Here's how the part is built. I have some questions about the finished solid (model axes, mm). A direction names the side the tool comes from. Round coordinates to 2 decimals unless told otherwise and drop trailing zeros. Loops run counter-clockwise (first coordinate to the right, second up) from the corner with the lowest first, then second, coordinate; pieces in that order, holes last. Notation, with made-up numbers: M 51.5,67.25 L 66.5,67.25 A19 cw 66.5,89.25 Z; hole C 53,79.5 d5. An arc over 180 degrees is marked long. Use a Markdown table: item, result.
```python
from build123d import *

# Parameters (mm, degrees)
BOSS_EXTRUDE1_DEPTH     = 12.7
SKETCH3_W               = 102.447825146
SKETCH3_H               = 31.827107341
BOSS_EXTRUDE2_DEPTH     = 88.9
SKETCH4_R               = 63.5
PILOT_DIA_DEPTH         = 3.175
F_1_2_20_TAPPED_HOLE2_D = 11.50874
CIRPATTERN2_COUNT       = 4


with BuildPart() as part:
    # Sketch1 → Base-Revolve (revolve)
    with BuildSketch(Plane.XY, mode=Mode.PRIVATE) as base_revolve_sk:
        with BuildLine():
            Line((0, 0), (0, 12.7))
            Line((0, 12.7), (-50.8, 12.7))
            Line((-50.8, 12.7), (-50.8, 69.85))
            Line((-50.8, 69.85), (-266.7, 69.85))
            Line((-266.7, 69.85), (-266.7, 76.2))
            Line((-266.7, 76.2), (-279.4, 76.2))
            ThreePointArc((-279.4, 76.2), (-297.360512242, 68.760512242), (-304.8, 50.8))
            Line((-304.8, 50.8), (-304.8, 0))
            Line((-304.8, 0), (0, 0))
        make_face()
    revolve(base_revolve_sk.sketch.rotate(Axis((0, 0, 0), (1, 0, 0)), 90), axis=Axis((0, 0, 0), (1, 0, 0)))

    # Sketch2 → Boss-Extrude1 (add)
    with BuildSketch(Plane(origin=(-50.8, 0, 0), x_dir=(0, 0, -1), z_dir=(1, 0, 0))):
        with BuildLine():
            Line((74.6125, -58.7375), (74.6125, 58.7375))
            ThreePointArc((74.6125, 58.7375), (69.962820151, 69.962820151), (58.7375, 74.6125))
            Line((58.7375, 74.6125), (-58.7375, 74.6125))
            ThreePointArc((-58.7375, 74.6125), (-69.962820151, 69.962820151), (-74.6125, 58.7375))
            Line((-74.6125, 58.7375), (-74.6125, -58.7375))
            ThreePointArc((-74.6125, -58.7375), (-69.962820151, -69.962820151), (-58.7375, -74.6125))
            Line((-58.7375, -74.6125), (58.7375, -74.6125))
            ThreePointArc((58.7375, -74.6125), (69.962820151, -69.962820151), (74.6125, -58.7375))
        make_face()
    extrude(amount=-BOSS_EXTRUDE1_DEPTH)

    # Sketch3 → Boss-Extrude2 (add)
    with BuildSketch(Plane(origin=(-203.2, 0, 0), x_dir=(0, 0, -1), z_dir=(1, 0, 0))):
        with Locations((0, 72.327654574)):
            Rectangle(SKETCH3_W, SKETCH3_H)
    extrude(amount=-BOSS_EXTRUDE2_DEPTH)

    # Sketch4 → pilot dia (add)
    with BuildSketch(Plane(origin=(-50.8, 0, 0), x_dir=(0, 0, -1), z_dir=(1, 0, 0))):
        with Locations(Location((0, 0, 0), (0, 0, 180))):
            Circle(SKETCH4_R)
    extrude(amount=PILOT_DIA_DEPTH)

    # 1/2-20 Tapped Hole2 (through all)
    with Locations(Plane.ZY.offset(63.5)):
        with Locations((58.7375, 58.7375)):
            f_1_2_20_tapped_hole2 = Hole(F_1_2_20_TAPPED_HOLE2_D / 2)

    # CirPattern2: 1/2-20 Tapped Hole2 ×4 about axis
    cirpattern2_axis = Axis((0, 0, 0), (1, 0, 0))
    for i in range(1, CIRPATTERN2_COUNT):
        add(f_1_2_20_tapped_hole2.rotate(cirpattern2_axis, i * 360 / CIRPATTERN2_COUNT), mode=Mode.SUBTRACT)


solid = part.part
```
Q1. Imagine slicing it at D-D, the plane x = -155. Please give me the cut outline in (y, z), then the cut area to 3 significant figures.
Return value:
| item | result |
|---|---|
| outline | C 0,0 d139.7 |
| area | 15,300 mm^2 |
Q2. For faces 4 (the flat face through (-247, 72, 51.224)), 5 (the cylindrical face through (-49.23, 61.99, -13.77)), 6 (the flat face through (-63.5, -49, 50)), 7 (the flat face through (-203.2, 76, 1)), which set-ups out of +Z, -Z, +X, -X, +Y, -Y let a thin tool reach every point of the face, with its end or its side?
Return value:
| item | result |
|---|---|
| face 4 | +Z, -X, +Y |
| face 5 | +X |
| face 6 | none |
| face 7 | +Y |
Q3. Will these pins go through, and if not, where does the flat tip stop? P1, Ø9.5, axis at y = 74, z = 19.5, coming from the +X side; P2, Ø4, axis at x = -56, z = -4, coming from the +Y side; P3, Ø14, axis at x = -55, y = -27.5, coming from the -Z side.
Return value:
| item | result |
|---|---|
| P1 | stops at x = -50.8 |
| P2 | stops at y = 74.61 |
| P3 | stops at z = -74.61 |
Q4. We'd pull the mould along Z, two halves only. Please class faces 1 (the cylindrical face through (-57.061, -59.487, 64.443)), 2 (the flat face through (0, 0, 0)), 3 (the flat face through (-247, 72, -51.224)): pulls with the +Z half, pulls with the -Z half, needs draft (parallel to the pull), parting line crosses it, or undercut.
Return value:
| item | result |
|---|---|
| face 1 | undercut |
| face 2 | needs draft |
| face 3 | pulls with the -Z half |
Q5. Imagine slicing it at B-B, the plane x = -223.5. Please give me the cut outline in (y, z), then the cut area to 3 significant figures.
Return value:
| item | result |
|---|---|
| outline | M 56.41,-51.22 L 88.24,-51.22 L 88.24,51.22 L 56.41,51.22 L 56.41,41.19 A69.85 ccw long 56.41,-41.19 Z |
| area | 17,800 mm^2 |
Q6. I need wall thicknesses on line 1 (X direction, y = 73.5, z = 4); line 2 (X direction, y = -16.5, z = -46) (3 decimals); line 3 (Z direction, x = -286, y = 69.5). Which ranges of each line are inside material? Lowest first, please. Write a range as from..to.
Return value:
| item | result |
|---|---|
| line 1 | x = -292.1..-203.2, -63.5..-50.8 |
| line 2 | x = -304.8..-47.625 |
| line 3 | z = -51.22..51.22 |
